Could you check a few things on this model? Use its own coordinates, in mm. A direction names the side the tool comes from. Round coordinates to 2 decimals unless told otherwise and drop trailing zeros. Loops run counter-clockwise (first coordinate to the right, second up) from the corner with the lowest first, then second, coordinate; pieces in that order, holes last. Notation, with made-up numbers: (-16.75, 66) - (31.25, 66) arc R28 ccw to (31.25, 91) - close; hole circle Ø6 at (3, -34.75). An arc over 180 degrees is marked (long way). Answer as CSV lines item,"result". Start each with the question number.
1) Which directions (+Z, -Z, +X, -X, +Y, -Y) give clear straight access to the entire face, cutting with the end or side of a thin tool? Please do faces 4 (the face through (0, -8.05, 3)), 5 (the face through (-0.54, -2.44, 9.04)).
2) Suppose I cut it at C-C, the plane y = -1.25. Write out the boundary of the cut face in (x, z), then the cut area to 3 significant figures.
3) Suppose I cut it at D-D, the plane x = -2.25. Write out the boundary of the cut face in (y, z).
4) Please list where these lines run through material, in increasing order: line 1 along X through (y, z) = (-9.25, 0); line 2 along Y through (x, z) = (0.75, 4); line 3 along Z through (x, y) = (-0.5, 4.5).
5) We'd pull the mould along X, two halves only. Please class faces 1 (the face through (0, -3, 10)), 2 (the face through (-2.44, -9.01, -0.54)), 3 (the face through (7.5, -6.2, 8.4)): pulls with the +X half, pulls with the -X half, needs draft (parallel to the pull), parting line crosses it, or undercut.
6) Suppose I cut it at A-A, the plane z = 2. Write out the boundary of the cut face in (x, y), then the cut area to 3 significant figures.
7) I'm going to push flat-ended pins straight in: pin 1 Ø3 at (x, z) = (-6, 4) entering from +Y; pin 2 Ø1.5 at (x, y) = (-2, -6.5) entering from -Z; pin 3 Ø3 at (x, y) = (4.5, -4.5) entering from -Z. Where does each tip first touch, or does it pass through?
8) Suppose I cut it at B-B, the plane x = 0. Write out the boundary of the cut face in (y, z).
```python
from build123d import *

# Parameters (mm, degrees)
RESSALTO_EXTRUS_O1_DEPTH  = 7.5
CONVERTER_S_LIDO1_START   = -7.5
CONVERTER_S_LIDO1_DEPTH   = 15
CONVERTER_S_LIDO1_2_DEPTH = 15
ESBO_O6_R                 = 2.5
CORTE_EXTRUS_O1_DEPTH     = 2
ESBO_O7_R                 = 2.5
CORTE_EXTRUS_O2_DEPTH     = 2


# Read off the part's stored shape, not the designer's step: Converter-Sólido1
with BuildPart() as part:
    # Esboço1 → Ressalto-extrusão1 (new, symmetric)
    with BuildSketch(Plane(origin=(0, 0, 0), x_dir=(0, 0, -1), z_dir=(1, 0, 0))):
        Polygon((-8, 10), (-8, -8), (10, -8), (10, -10), (-10, -10), (-10, 10), align=None)
    extrude(amount=RESSALTO_EXTRUS_O1_DEPTH, both=True)

    # Converter-Sólido1 outline → Converter-Sólido1 (cut)
    with BuildSketch(Plane.YZ.offset(CONVERTER_S_LIDO1_START)):
        with BuildLine():
            Line((-10, 10), (-10, 7.24))
            ThreePointArc((-10, 7.24), (-9.191614716, 9.191614716), (-7.24, 10))
            Line((-7.24, 10), (-10, 10))
        make_face()
        with BuildLine():
            Line((-8.05, 7.24), (-8.05, -10))
            Line((-8.05, -10), (-8, -10))
            Line((-8, -10), (-8, 7.520178515))
            ThreePointArc((-8, 7.520178515), (-8.037402032, 7.382302495), (-8.05, 7.24))
        make_face()
        with BuildLine():
            Line((10, 8), (10, 8.05))
            Line((10, 8.05), (-7.24, 8.05))
            ThreePointArc((-7.24, 8.05), (-7.382302495, 8.037402032), (-7.520178515, 8))
            Line((-7.520178515, 8), (10, 8))
        make_face()
    extrude(amount=CONVERTER_S_LIDO1_DEPTH, mode=Mode.SUBTRACT)

    # Converter-S_lido1 2 outline → Converter-S_lido1 2 (add)
    with BuildSketch(Plane.YZ.offset(CONVERTER_S_LIDO1_START)):
        with BuildLine():
            Line((-8, 8), (-8, 7.520178515))
            ThreePointArc((-8, 7.520178515), (-7.812756493, 7.812756493), (-7.520178515, 8))
            Line((-7.520178515, 8), (-8, 8))
        make_face()
    extrude(amount=CONVERTER_S_LIDO1_2_DEPTH)

    # Esboço6 → Corte-extrusão1 (cut)
    with BuildSketch(Plane.XY.offset(10)):
        Circle(ESBO_O6_R)
        with BuildLine():
            Line((-7.5, 0), (-7.5, 10))
            Line((-7.5, 10), (7.5, 10))
            Line((7.5, 10), (7.5, 0))
            ThreePointArc((7.5, 0), (0, 7.5), (-7.5, 0))
        make_face()
    extrude(amount=-CORTE_EXTRUS_O1_DEPTH, mode=Mode.SUBTRACT)

    # Esboço7 → Corte-extrusão2 (cut)
    with BuildSketch(Plane(origin=(0, -8.05, 0), x_dir=(1, 0, 0), z_dir=(0, 1, 0))):
        with Locations(Location((0, 0, 0), (0, 0, 270))):
            Circle(ESBO_O7_R)
        with BuildLine():
            Line((7.5, 0), (7.5, 10))
            Line((7.5, 10), (-7.5, 10))
            Line((-7.5, 10), (-7.5, 0))
            ThreePointArc((-7.5, 0), (0, 7.5), (7.5, 0))
        make_face()
    extrude(amount=-CORTE_EXTRUS_O2_DEPTH, mode=Mode.SUBTRACT)


solid = part.part
```
Filled sheet:
1,face 4,"-Z, +X, -X, +Y"
1,face 5,"+Z, -Z"
2,outline,"(-7.5, 8.05) - (-2.17, 8.05) - (-2.17, 10) - (-7.5, 10) - close; (2.17, 8.05) - (7.5, 8.05) - (7.5, 10) - (2.17, 10) - close"
2,area,"20.8 mm²"
3,outline,"(-10, -7.15) - (-8.05, -7.15) - (-8.05, -1.09) - (-10, -1.09) - close; (-10, 1.09) - (-8.05, 1.09) - (-8.05, 7.24) arc R0.81 cw to (-7.24, 8.05) - (-1.09, 8.05) - (-1.09, 10) - (-7.24, 10) arc R2.76 ccw to (-10, 7.24) - close; (1.09, 8.05) - (7.15, 8.05) - (7.15, 10) - (1.09, 10) - close"
4,line 1,"-7.5 to -2.5, 2.5 to 7.5"
4,line 2,"-10 to -8.05"
4,line 3,"8.05 to 10"
5,face 1,"needs draft"
5,face 2,"undercut"
5,face 3,"pulls with the +X half"
6,outline,"(-7.5, -10) - (-1.5, -10) - (-1.5, -8.05) - (-7.5, -8.05) - close; (1.5, -10) - (7.5, -10) - (7.5, -8.05) - (1.5, -8.05) - close"
6,area,"23.4 mm²"
7,pin 1,"y = -8.05"
7,pin 2,"z = 8.05"
7,pin 3,"z = 8.05"
8,outline,"(-10, -7.5) - (-8.05, -7.5) - (-8.05, -2.5) - (-10, -2.5) - close; (-10, 2.5) - (-8.05, 2.5) - (-8.05, 7.24) arc R0.81 cw to (-7.24, 8.05) - (-2.5, 8.05) - (-2.5, 10) - (-7.24, 10) arc R2.76 ccw to (-10, 7.24) - close; (2.5, 8.05) - (7.5, 8.05) - (7.5, 10) - (2.5, 10) - close"
